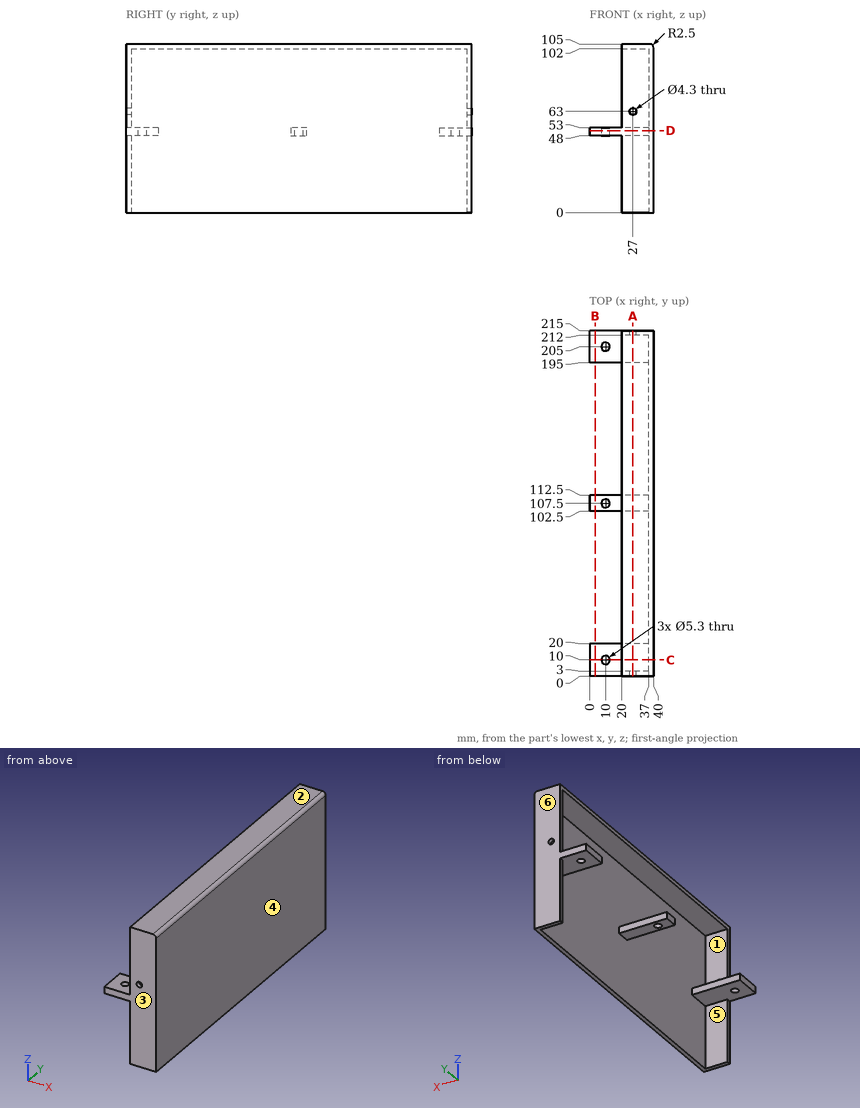
Print and shaded views of the part. All mm, measured from the part's lowest x, y and z. A direction names the side the tool comes from. Round coordinates to 2 decimals unless told otherwise and drop trailing zeros. Write each loop counter-clockwise with the first axis right and the second up, starting at its lowest first coordinate (ties: lowest second). Pieces come first, ordered by that corner, then holes. Notation, with made-up numbers: (-17.5, -14) -> (20.5, -14) arc R16 cw to (20.5, -9) -> close; hole circle Ø2 at (-18, 67.25). An arc over 180 degrees is marked (long way). Answer in a Markdown table with one row per item. Add a question column.
Item 1: Saw through at D-D, the plane z = 51. Write the cut outline in (x, y), then the cut area to 3 significant figures.
Item 2: Drill centre lines: line 1 (Y direction, x = 10, z = 51.45); line 2 (X direction, y = 212.85, z = 63); line 3 (Y direction, x = 25.5, z = 35.5). Where is each one in solid material? Low to high. Write a range as from..to.
Item 3: Mould opens along Y. For the marked faces 3, 4, 5 and 6 say: pulls with the +Y half, pulls with the -Y half, needs draft (parallel to the pull), parting line crosses it, or undercut.
Item 4: Saw through at C-C, the plane y = 10. Write the cut outline in (x, z).
Item 5: Which spindle directions (+Z, -Z, +X, -X, +Y, -Y) get a long thin tool onto all of the face, cutting with end or side? Do the marked faces 1 and 2. Say none if no direction does.
Item 6: Saw through at B-B, the plane x = 3.5. Write the cut outline in (y, z).
Item 7: Drop flat-ended pins along their axis: pin 1 Ø16 at (x, y) = (11.5, 209.5) entering from +Z; pin 2 Ø3.5 at (x, z) = (27, 63) entering from +Y; pin 3 Ø3 at (y, z) = (158.5, 82.5) entering from -X; pin 4 Ø8 at (x, y) = (19, 135) entering from -Z. Give the stop position or say it passes through.
Item 8: Saw through at A-A, the plane x = 27. Write the cut outline in (y, z), then the cut area to 3 significant figures.
Findings below:
| question | item | result |
|---|---|---|
| 1 | outline | (0, 0) -> (40, 0) -> (40, 215) -> (0, 215) -> (0, 195) -> (37, 195) -> (37, 112.5) -> (0, 112.5) -> (0, 102.5) -> (37, 102.5) -> (37, 20) -> (0, 20) -> close; hole circle Ø5.3 at (10, 10); hole circle Ø5.3 at (10, 107.5); hole circle Ø5.3 at (10, 205) |
| 1 | area | 2,430 mm^2 |
| 2 | line 1 | y = 0..7.35, 12.65..20, 102.5..104.85, 110.15..112.5, 195..202.35, 207.65..215 |
| 2 | line 2 | x = 20..24.85, 29.15..40 |
| 2 | line 3 | y = 0..3, 212..215 |
| 3 | face 3 | pulls with the -Y half |
| 3 | face 4 | needs draft |
| 3 | face 5 | undercut |
| 3 | face 6 | pulls with the +Y half |
| 4 | outline | (0, 48) -> (7.35, 48) -> (7.35, 53) -> (0, 53) -> close; (12.65, 48) -> (37, 48) -> (37, 0) -> (40, 0) -> (40, 102.5) arc R2.5 ccw to (37.5, 105) -> (20, 105) -> (20, 102) -> (37, 102) -> (37, 53) -> (12.65, 53) -> close |
| 5 | face 1 | -X |
| 5 | face 2 | +Z, +X, -X, +Y, -Y |
| 6 | outline | (0, 48) -> (20, 48) -> (20, 53) -> (0, 53) -> close; (102.5, 48) -> (112.5, 48) -> (112.5, 53) -> (102.5, 53) -> close; (195, 48) -> (215, 48) -> (215, 53) -> (195, 53) -> close |
| 7 | pin 1 | stops at z = 53 |
| 7 | pin 2 | passes through |
| 7 | pin 3 | stops at x = 37 |
| 7 | pin 4 | stops at z = 102 |
| 8 | outline | (0, 0) -> (3, 0) -> (3, 48) -> (20, 48) -> (20, 53) -> (3, 53) -> (3, 60.85) -> (0, 60.85) -> close; (0, 65.15) -> (3, 65.15) -> (3, 102) -> (212, 102) -> (212, 65.15) -> (215, 65.15) -> (215, 105) -> (0, 105) -> close; (102.5, 48) -> (112.5, 48) -> (112.5, 53) -> (102.5, 53) -> close; (195, 48) -> (212, 48) -> (212, 0) -> (215, 0) -> (215, 60.85) -> (212, 60.85) -> (212, 53) -> (195, 53) -> close |
| 8 | area | 1,450 mm^2 |
